```python
from build123d import *

# Parameters (mm, degrees)
BOX_W           = 52
BOX_H           = 38
BOX_DEPTH       = 16.1
SKETCH003_R     = 4.2
SKETCH003_W     = 19
SKETCH003_H     = 10
POCKET_DEPTH    = 38.001
SKETCH007_R     = 1.4
POCKET001_DEPTH = 16.101
SKETCH008_R     = 1.5
POCKET002_DEPTH = 3
SKETCH004_R     = 1.5
POCKET003_DEPTH = 3
SKETCH013_R     = 1.68
POCKET004_DEPTH = 16.101
FILLET004_R     = 5


with BuildPart() as part:
    # Box → Box (new body)
    with BuildSketch(Plane.XY):
        with Locations((26, 19)):
            Rectangle(BOX_W, BOX_H)
    extrude(amount=BOX_DEPTH)

    # Sketch003 → Pocket (cut, through all)
    with BuildSketch(Plane(origin=(0, 38, 0), x_dir=(-1, 0, 0), z_dir=(0, 1, 0))):
        with Locations((-46, 8.25)):
            Circle(SKETCH003_R)
        with Locations((-6, 8.25)):
            Circle(SKETCH003_R)
        with Locations((-26, 8.1)):
            Rectangle(SKETCH003_W, SKETCH003_H)
    extrude(amount=-POCKET_DEPTH, mode=Mode.SUBTRACT)

    # Sketch007 → Pocket001 (cut, through all)
    with BuildSketch(Plane.XY.offset(16.1)):
        with Locations((13, 5)):
            Circle(SKETCH007_R)
        with Locations((39, 5)):
            Circle(SKETCH007_R)
        with Locations((39, 33)):
            Circle(SKETCH007_R)
        with Locations((13, 33)):
            Circle(SKETCH007_R)
    extrude(amount=-POCKET001_DEPTH, mode=Mode.SUBTRACT)

    # Sketch008 → Pocket002 (cut)
    with BuildSketch(Plane(origin=(0, 0, 0), x_dir=(0, -1, 0), z_dir=(-1, 0, 0))):
        with Locations((-29.5, 8.25)):
            Circle(SKETCH008_R)
        with Locations((-9.5, 8.25)):
            Circle(SKETCH008_R)
    extrude(amount=-POCKET002_DEPTH, mode=Mode.SUBTRACT)

    # Sketch004 → Pocket003 (cut)
    with BuildSketch(Plane.YZ.offset(52)):
        with Locations((9.5, 8.25)):
            Circle(SKETCH004_R)
        with Locations((29.5, 8.25)):
            Circle(SKETCH004_R)
    extrude(amount=-POCKET003_DEPTH, mode=Mode.SUBTRACT)

    # Sketch013 → Pocket004 (cut, through all)
    with BuildSketch(Plane.XY.offset(16.1)):
        with Locations((26, 4)):
            Circle(SKETCH013_R)
    extrude(amount=-POCKET004_DEPTH, mode=Mode.SUBTRACT)

    # Fillet004
    fillet004_edges = [part.edges().sort_by_distance(p)[0] for p in [
        (52, 19, 16.1),
        (52, 19, 0),
        (0, 19, 16.1),
        (0, 19, 0),
    ]]
    fillet(fillet004_edges, radius=FILLET004_R)


solid = part.part
```
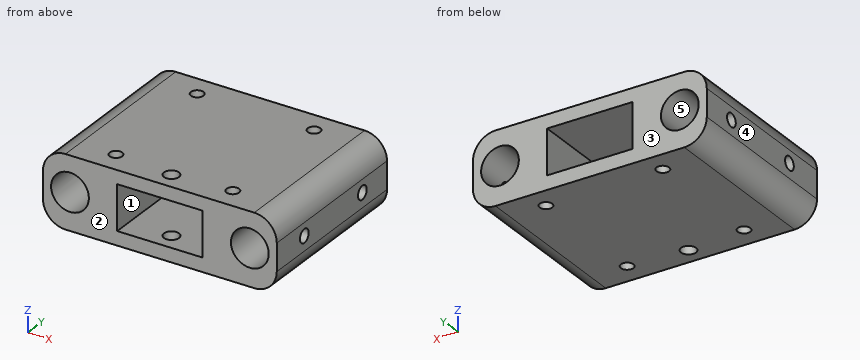
Geometry: final body of the model. Coordinates: model frame, mm. Face numbers are marked on the shaded views. A direction names the side the tool comes from. Round coordinates to 2 decimals unless told otherwise and drop trailing zeros. Write each loop counter-clockwise with the first axis right and the second up, starting at its lowest first coordinate (ties: lowest second). Pieces come first, ordered by that corner, then holes.
Item 1: Set-up query: the marked faces 1 and 2. Return all of +Z, -Z, +X, -X, +Y, -Y with unobstructed straight access to the full face (end or side cutting, diameter ignored); none if empty.
Item 2: Section query D-D (z = 15). Return loops of the section in (x, y), plus the area to 3 significant figures.
Item 3: Section query C-C (y = 17). Return loops of the section in (x, z), plus the area to 3 significant figures.
Item 4: Mould query, pull axis X, two halves, no side actions, for the marked faces 3, 4 and 5. Classes: +X half, -X half, draft (parallel to the pull), parting line (faces both ways), or undercut.
Item 5: Pin query (flat end, axial travel): P1, Ø4.5, axis at x = 26, y = 4, coming from the -Z side; P2, Ø1.7, axis at x = 13, y = 5, coming from the +Z side; P3, Ø2, axis at y = 25.5, z = 12.5, coming from the -X side; P4, Ø2.5, axis at y = 9.5, z = 8.25, coming from the +X side. Return the tip coordinate at first contact, or that it passes through.
Item 6: Section query A-A (x = 39). Return loops of the section in (y, z), plus the area to 3 significant figures.
Item 7: Section query B-B (x = 18). Return loops of the section in (y, z).
Item 8: Material intervals for L1, parallel to Y at x = 26, z = 2.4; L2, parallel to Z at x = 26.5, y = 16; L3, parallel to X at y = 29, z = 9.75, sorted ascending.
Completed:
1. face 1: +Y, -Y
1. face 2: +Z, -Z, +X, -X, -Y
2. outline: (1.87, 0) - (50.13, 0) - (50.13, 38) - (1.87, 38) - close; hole circle Ø2.8 at (13, 5); hole circle Ø2.8 at (13, 33); hole circle Ø3.36 at (26, 4); hole circle Ø2.8 at (39, 5); hole circle Ø2.8 at (39, 33)
2. area: 1,800 mm2
3. outline: (0, 5) arc R5 ccw to (5, 0) - (47, 0) arc R5 ccw to (52, 5) - (52, 11.1) arc R5 ccw to (47, 16.1) - (5, 16.1) arc R5 ccw to (0, 11.1) - close; hole circle Ø8.4 at (6, 8.25); hole (16.5, 3.1) - (35.5, 3.1) - (35.5, 13.1) - (16.5, 13.1) - close; hole circle Ø8.4 at (46, 8.25)
3. area: 515 mm2
4. face 3: draft
4. face 4: -X half
4. face 5: undercut
5. P1: stops at z = 0
5. P2: passes through
5. P3: stops at x = 0.02
5. P4: stops at x = 41.99
6. outline: (0, 0) - (3.6, 0) - (3.6, 16.1) - (0, 16.1) - close; (6.4, 0) - (31.6, 0) - (31.6, 16.1) - (6.4, 16.1) - close; (34.4, 0) - (38, 0) - (38, 16.1) - (34.4, 16.1) - close
6. area: 522 mm2
7. outline: (0, 0) - (38, 0) - (38, 3.1) - (0, 3.1) - close; (0, 13.1) - (38, 13.1) - (38, 16.1) - (0, 16.1) - close
8. L1: y = 0 to 2.32, 5.68 to 38
8. L2: z = 0 to 3.1, 13.1 to 16.1
8. L3: x = 0 to 2.08, 9.92 to 16.5, 35.5 to 42.08, 49.92 to 52
